Geometry check sheet. Reference: drawing and pictorial views, mm from the part's lowest x, y, z. Coordinates: 2 decimals unless noted, no trailing zeros. Loops run counter-clockwise (first coordinate to the right, second up) from the corner with the lowest first, then second, coordinate; pieces in that order, holes last. Notation, with made-up numbers: (40, 13.25) - (97, 13.25) arc R33 cw to (97, 52.25) - close; hole circle Ø7 at (37.25, -0.5). An arc over 180 degrees is marked (long way). Use a Markdown table: item, result. Add a question column.
1) Sectioned sample at A-A, the plane z = 26.5. Enter the section's corners in (x, y).
2) Thickness scan on line 1 (Z direction, x = 9, y = 3); line 2 (Z direction, x = 58, y = 5.5); line 3 (X direction, y = 4.75, z = 31). Record the ranges inside material, lowest first.
3) Sectioned sample at D-D, the plane y = 2. Enter the section's corners in (x, z), then the cut area to 3 significant figures.
4) Sectioned sample at B-B, the plane z = 16. Enter the section's corners in (x, y), then the cut area to 3 significant figures.
5) Sectioned sample at C-C, the plane x = 9. Enter the section's corners in (y, z).
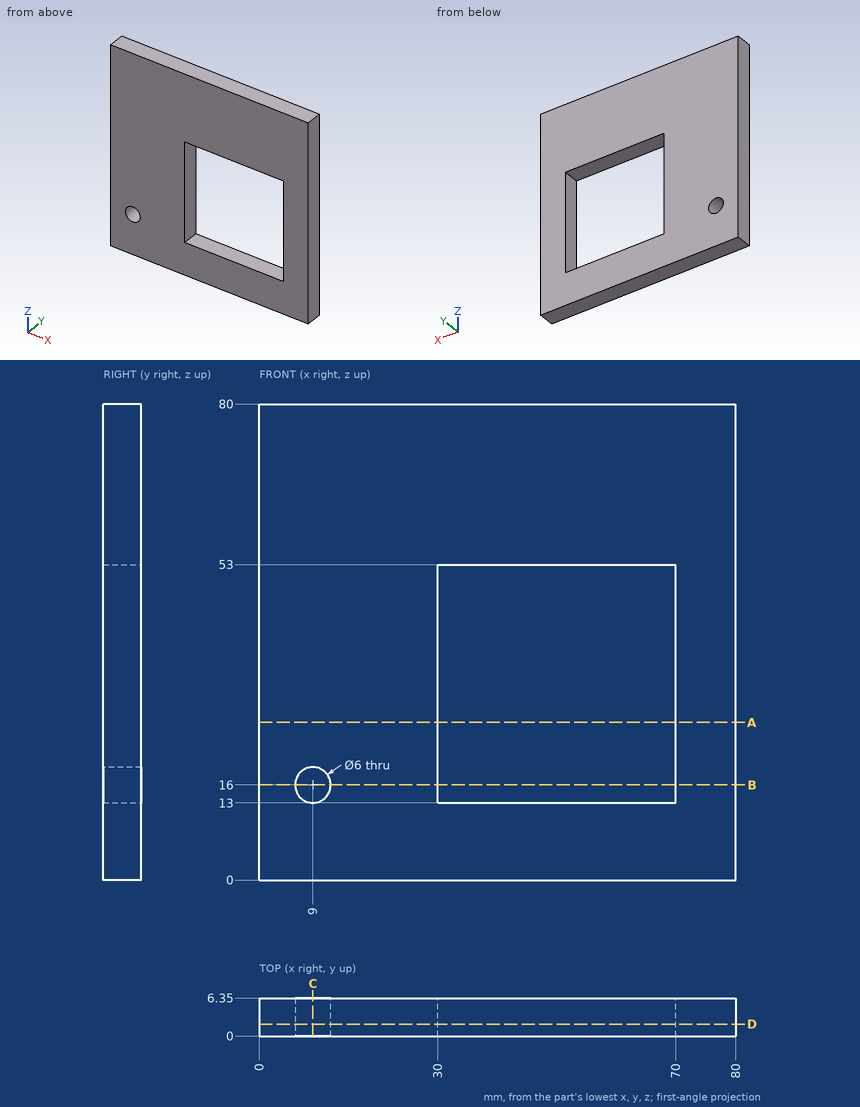
Solved:
| question | item | result |
|---|---|---|
| 1 | outline | (0, 0) - (30, 0) - (30, 6.35) - (0, 6.35) - close; (70, 0) - (80, 0) - (80, 6.35) - (70, 6.35) - close |
| 2 | line 1 | z = 0 to 13, 19 to 80 |
| 2 | line 2 | z = 0 to 13, 53 to 80 |
| 2 | line 3 | x = 0 to 30, 70 to 80 |
| 3 | outline | (0, 0) - (80, 0) - (80, 80) - (0, 80) - close; hole circle Ø6 at (9, 16); hole (30, 13) - (70, 13) - (70, 53) - (30, 53) - close |
| 3 | area | 4,770 mm2 |
| 4 | outline | (0, 0) - (6, 0) - (6, 6.35) - (0, 6.35) - close; (12, 0) - (30, 0) - (30, 6.35) - (12, 6.35) - close; (70, 0) - (80, 0) - (80, 6.35) - (70, 6.35) - close |
| 4 | area | 216 mm2 |
| 5 | outline | (0, 0) - (6.35, 0) - (6.35, 13) - (0, 13) - close; (0, 19) - (6.35, 19) - (6.35, 80) - (0, 80) - close |
